Part model, mm, in its own coordinate system. A direction names the side the tool comes from. Coordinates: 2 decimals unless noted, no trailing zeros. Loops run counter-clockwise (first coordinate to the right, second up) from the corner with the lowest first, then second, coordinate; pieces in that order, holes last. Notation, with made-up numbers: (-4.5, 48.25) -> (22.5, 48.25) arc R20 ccw to (22.5, 70.25) -> close; hole circle Ø3 at (0, 1). An arc over 180 degrees is marked (long way). One line per item, written item: value. Start each with the question number.
from build123d import *

# Parameters (mm, degrees)
SKETCH31_R   = 25.5
SKETCH31_R_2 = 25


with BuildPart() as part:
    # Sweep1: sweep along a path in Sketch3
    with BuildLine(Plane(origin=(0, 0, 0), x_dir=(0, 0, -1), z_dir=(1, 0, 0))) as sweep1_path:
        Line((0, 0), (260, 0))
        ThreePointArc((260, 0), (288.284271247, -11.715728753), (300, -40))
        Line((300, -40), (300, -440))
        ThreePointArc((300, -440), (288.284271247, -468.284271247), (260, -480))
        Line((260, -480), (224.43, -480))
    # Sketch31 → Sweep1 (sweep)
    with BuildSketch(Plane.XY):
        Circle(SKETCH31_R)
        Circle(SKETCH31_R_2, mode=Mode.SUBTRACT)
    sweep(path=sweep1_path.line)


solid = part.part
1) Slice it at A-A (x = 0). Give the cut face in (y, z).
2) Pin check, flat tips, straight feed: pin 1 Ø1.5 at (x, z) = (-18.5, -201.5) entering from -Y; pin 2 Ø3 at (x, z) = (17, -126.5) entering from +Y; pin 3 Ø5 at (x, y) = (-18.5, -234.5) entering from +Z. Stop position of each tip, or through.
3) Slice it at C-C (z = -203). Give the cut face in (x, y).
4) Tool access for faces 3 (the cylindrical face through (-5.5, 24.9, -131.8)), 4 (the flat face through (-18.8, -496.9, -224.43)), 5 (the cylindrical face through (-3.255, -242.8, -275.213)): list every direction of +Z, -Z, +X, -X, +Y, -Y with a clear straight run to the whole face (end or side of a thin tool).
5) Pull direction Y, two halves, no side cores. Call faces 1 (the cylindrical face through (23.846, -7.509, -131.82)), 2 (the flat face through (16.9, -18.8, 0)): +Y half, -Y half, draft (parallel to the pull), parting line (faces both ways), or undercut.
6) Slice it at B-B (y = -243). Give the cut face in (x, z), then the cut area to 3 significant figures.
7) Probe line 1 (Y direction, x = 0, z = -252); line 2 (Y direction, x = 0, z = -149); line 3 (Z direction, x = -1.5, y = -251). List the from-to ranges inside material, lowest first. Write a range as from..to.
Check sheet entries:
1. outline: (-505.5, -260) arc R65.5 ccw to (-440, -325.5) -> (-40, -325.5) arc R65.5 ccw to (25.5, -260) -> (25.5, 0) -> (25, 0) -> (25, -260) arc R65 cw to (-40, -325) -> (-440, -325) arc R65 cw to (-505, -260) -> (-505, -224.43) -> (-505.5, -224.43) -> close; (-455, -260) arc R15 ccw to (-440, -275) -> (-40, -275) arc R15 ccw to (-25, -260) -> (-25, 0) -> (-25.5, 0) -> (-25.5, -260) arc R14.5 cw to (-40, -274.5) -> (-440, -274.5) arc R14.5 cw to (-454.5, -260) -> (-454.5, -224.43) -> (-455, -224.43) -> close
2. pin 1: stops at y = -18.31
2. pin 2: stops at y = 20.25
2. pin 3: stops at z = -280.14
3. outline: circle Ø51 at (0, 0); hole circle Ø50 at (0, 0)
4. face 3: +Z
4. face 4: +Z, +X, -X, -Y
4. face 5: none
5. face 1: undercut
5. face 2: draft
6. outline: circle Ø51 at (0, -300); hole circle Ø50 at (0, -300)
6. area: 79.3 mm^2
7. line 1: y = -505.5..-505, -455..-454.5, -25.5..-25, 25..25.5
7. line 2: y = -25.5..-25, 25..25.5
7. line 3: z = -325.46..-324.95, -275.05..-274.54
